Source: CAD feature listing. Evaluate the final solid. Frame: model axes, mm. A direction names the side the tool comes from. Give positions to 0.01 mm unless a question says otherwise; leave off trailing zeros. Write each loop counter-clockwise with the first axis right and the second up, starting at its lowest first coordinate (ties: lowest second). Pieces come first, ordered by that corner, then holes. Notation, with made-up numbers: (44, -2) -> (53, -2) arc R16 cw to (53, 3) -> close; hole circle Ø1 at (17.5, 15.5). An arc over 180 degrees is marked (long way). Write item = value, one per line.
from build123d import *

# Parameters (mm, degrees)
BASPROSKE_W     = 30
BASPROSKE_H     = 55
TOOTHCUT_DEPTH  = 84.366660003
TEETHCUTS_COUNT = 20
TEETHCUTS_ANGLE = 342
BORSKE_R        = 2.5
BORE_DEPTH      = 50.0000508
SKETCH_1_R      = 2
EXTRUDE_1_DEPTH = 10


with BuildPart() as part:
    # BasProSke → Base-Revolve (revolve)
    with BuildSketch(Plane(origin=(0, 0, 0), x_dir=(1, 0, 0), z_dir=(0, 1, 0)), mode=Mode.PRIVATE) as base_revolve_sk:
        with Locations((15, 27.5)):
            Rectangle(BASPROSKE_W, BASPROSKE_H)
    revolve(base_revolve_sk.sketch.rotate(Axis((-10, 0, 0), (1, 0, 0)), 180), axis=Axis((-10, 0, 0), (1, 0, 0)))

    # TooCutSke → ToothCut (cut, through all)
    with BuildSketch(Plane(origin=(0, 0, 0), x_dir=(0, 0, -1), z_dir=(1, 0, 0))):
        with BuildLine():
            ThreePointArc((2.464838288, 43.679509764), (0, 43.749), (-2.464838288, 43.679509764))
            ThreePointArc((-2.464838288, 43.679509764), (-4.057398861, 49.476814676), (-7.300899231, 54.538899105))
            ThreePointArc((-7.300899231, 54.538899105), (0, 55.0254), (7.300899231, 54.538899105))
            ThreePointArc((7.300899231, 54.538899105), (4.057398861, 49.476814676), (2.464838288, 43.679509764))
        make_face()
    toothcut = extrude(amount=TOOTHCUT_DEPTH, mode=Mode.SUBTRACT)

    # TeethCuts: ToothCut ×20 about axis
    teethcuts_axis = Axis((-10, 0, 0), (1, 0, 0))
    for i in range(1, TEETHCUTS_COUNT):
        add(toothcut.rotate(teethcuts_axis, i * TEETHCUTS_ANGLE / (TEETHCUTS_COUNT - 1)), mode=Mode.SUBTRACT)

    # BorSke → Bore (cut, symmetric)
    with BuildSketch(Plane(origin=(0, 0, 0), x_dir=(0, 0, -1), z_dir=(1, 0, 0))):
        with Locations(Location((0, 0, 0), (0, 0, 180))):
            Circle(BORSKE_R)
    extrude(amount=BORE_DEPTH, both=True, mode=Mode.SUBTRACT)

    # 草图1 → 凸台-拉伸1 (add)
    with BuildSketch(Plane.ZY):
        with Locations(Location((0, -17.25, 0), (0, 0, 180))):
            Circle(SKETCH_1_R)
        with Locations(Location((-14.938938215, -8.625, 0), (0, 0, 180))):
            Circle(SKETCH_1_R)
        with Locations(Location((-14.938938215, 8.625, 0), (0, 0, 180))):
            Circle(SKETCH_1_R)
        with Locations(Location((0, 17.25, 0), (0, 0, 180))):
            Circle(SKETCH_1_R)
        with Locations(Location((14.938938215, 8.625, 0), (0, 0, 180))):
            Circle(SKETCH_1_R)
        with Locations(Location((14.938938215, -8.625, 0), (0, 0, 180))):
            Circle(SKETCH_1_R)
    extrude(amount=EXTRUDE_1_DEPTH)


solid = part.part
1) Contact query for flat-ended pins moving along their axis: pin 1 (1 mm diameter, centred on x = 6.5, y = -34.5, fed in from -Z); pin 2 (5 mm diameter, centred on x = 4, y = -28, fed in from +Z); pin 3 (12 mm diameter, centred on y = -10.5, z = -7, fed in from -X); pin 4 (6 mm diameter, centred on x = -5, z = 35.5, fed in from -Y). Output: stop coordinate, or through.
Computed:
pin_1 = -38.92
pin_2 = 48.73
pin_3 = 0
pin_4 = through
2) Draft query along Y for faces 1 (the cylindrical face through (14.79, -19.082, 45.727)), 2 (the cylindrical face through (14.79, -45.727, -19.082)), 3 (the cylindrical face through (14.79, 37.677, -32.424)). Return one class per face: pulls with the +Y half, pulls with the -Y half, needs draft (parallel to the pull), parting line crosses it, or undercut.
Computed:
face_1 = undercut
face_2 = pulls with the -Y half
face_3 = pulls with the +Y half
3) Access query for faces 4 (the cylindrical face through (14.79, -48.21, 11.44)), 5 (the cylindrical face through (-4.93, 8.54, -12.94)), 6 (the cylindrical face through (14.79, -37.593, -32.278)), 7 (the cylindrical face through (14.79, -4.086, -49.54)). Directions: +Z, -Z, +X, -X, +Y, -Y. A direction counts if a zero-diameter tool reaches every point of the face in a straight line with its end or side. Return the directions, or none.
Computed:
face_4 = +X, -X
face_5 = -X
face_6 = +X, -X, -Y
face_7 = -Z, +X, -X
4) Material intervals for L1, parallel to Z at x = 11.5, y = -48; L2, parallel to Y at x = 16, z = 44; L3, parallel to X at y = 17, z = 23, sorted ascending.
Computed:
L1 = -26.18 to -21.47, -11.46 to -3.47, 3.47 to 11.46, 21.47 to 26.18
L2 = -26.07 to -17.7, -11.42 to -2.51, 2.51 to 11.42, 17.7 to 26.07
L3 = 0 to 30
5) Cut plane C-C (y = 17.25). Return the cut outline in (x, z), then the cut area to 3 significant figures.
Computed:
outline = (-10, -2) -> (0, -2) -> (0, -43.33) -> (30, -43.33) -> (30, 43.33) -> (0, 43.33) -> (0, 2) -> (-10, 2) -> close
area = 2,640 mm²
6) Cut plane A-A (y = 0). Return the cut outline in (x, z), then the cut area to 3 significant figures.
Computed:
outline = (0, -43.75) -> (30, -43.75) -> (30, -2.5) -> (0, -2.5) -> close; (0, 2.5) -> (30, 2.5) -> (30, 43.75) -> (0, 43.75) -> close
area = 2,470 mm²
7) Cut plane B-B (z = 0). Return the cut outline in (x, y).
Computed:
outline = (-10, -19.25) -> (0, -19.25) -> (0, -43.75) -> (30, -43.75) -> (30, -2.5) -> (0, -2.5) -> (0, -15.25) -> (-10, -15.25) -> close; (-10, 15.25) -> (0, 15.25) -> (0, 2.5) -> (30, 2.5) -> (30, 43.75) -> (0, 43.75) -> (0, 19.25) -> (-10, 19.25) -> close
